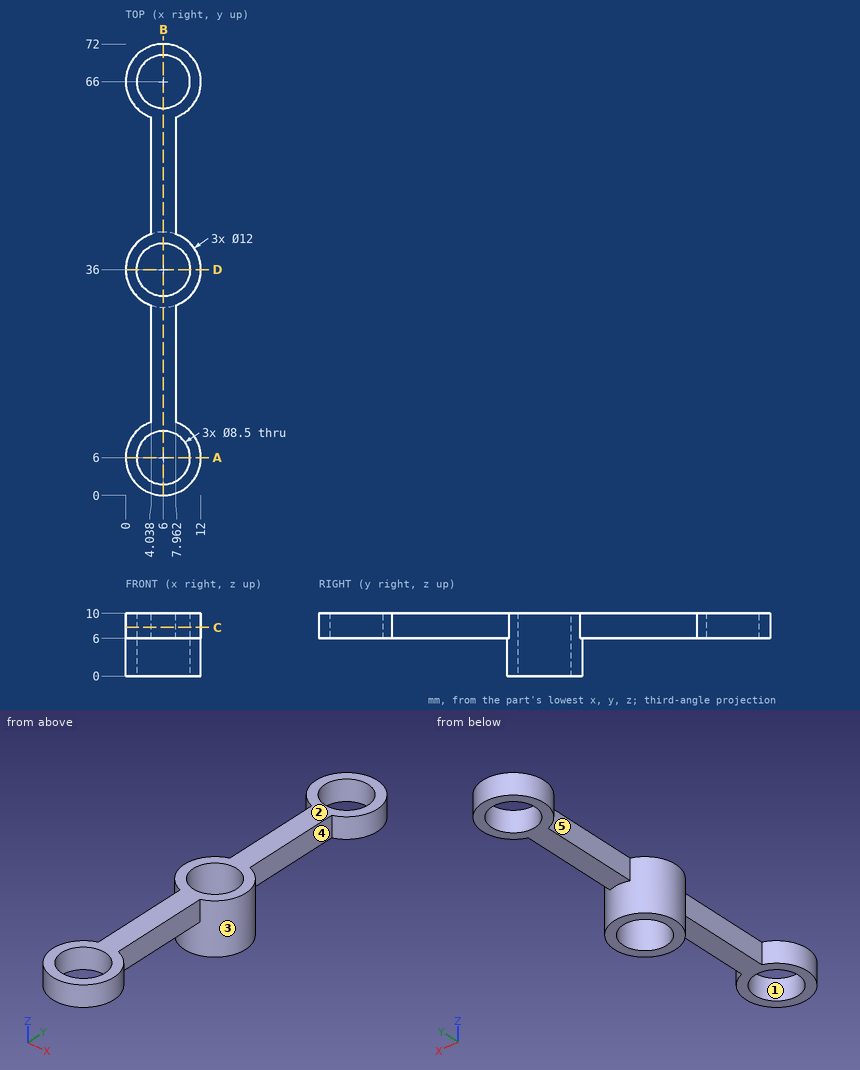
Geometry: see drawing. Coordinates: mm, zero at the bounding-box minimum. A direction names the side the tool comes from. Give positions to 0.01 mm unless a question says otherwise; leave off trailing zeros. Order: outer loops, then holes, each group sorted by start corner. A loop starts at its lowest first (then second) coordinate and runs counter-clockwise, first axis right, second up. Notation, with made-up numbers: M -27,65 L -18,65 A20 cw -18,93 Z; hole C 68.5,47 d4. An arc over 180 degrees is marked long. Answer as a JSON object with one key per item and string values.
1. Cut plane B-B, the plane x = 6. Output: boundary loops of the cut face in (y, z).
Result sheet:
{"outline": "M 0,6 L 1.75,6 L 1.75,10 L 0,10 Z; M 10.25,6 L 30,6 L 30,0 L 31.75,0 L 31.75,10 L 10.25,10 Z; M 40.25,0 L 42,0 L 42,6 L 61.75,6 L 61.75,10 L 40.25,10 Z; M 70.25,6 L 72,6 L 72,10 L 70.25,10 Z"}
2. Cut plane A-A, the plane y = 6. Output: boundary loops of the cut face in (x, z), and give its area (3 significant figures).
Result sheet:
{"outline": "M 0,6 L 1.75,6 L 1.75,10 L 0,10 Z; M 10.25,6 L 12,6 L 12,10 L 10.25,10 Z", "area": "14.0 mm²"}
3. Reachability of the marked faces 3, 4 and 5 from +Z, -Z, +X, -X, +Y, -Y: full face, straight path, thin tool, end or side. Return the list, or none.
Result sheet:
{"face 3": "-Z", "face 4": "+Z, -Z, +X", "face 5": "+Z, -Z, -X"}
4. Ray query, line 1 (X direction, y = 36, z = 4.75); line 2 (Y direction, x = 7.25, z = 7.5); line 3 (Z direction, x = 6.5, y = 59). Return the intervals inside material, ascending. Write a range as [from, to].
Result sheet:
{"line 1": "[0, 1.75], [10.25, 12]", "line 2": "[0.13, 1.94], [10.06, 31.94], [40.06, 61.94], [70.06, 71.87]", "line 3": "[6, 10]"}
5. Cut plane D-D, the plane y = 36. Output: boundary loops of the cut face in (x, z), and give its area (3 significant figures).
Result sheet:
{"outline": "M 0,0 L 1.75,0 L 1.75,10 L 0,10 Z; M 10.25,0 L 12,0 L 12,10 L 10.25,10 Z", "area": "35.0 mm²"}
6. First-contact query: P1, Ø2, axis at y = 25, z = 8.5, coming from the +X side; P2, Ø6, axis at x = 8.5, y = 19.5, coming from the -Z side; P3, Ø6, axis at x = 3, z = 4, coming from the -Y side. Flat tips, straight axial feed; report the tip coordinate or a pass-through.
Result sheet:
{"P1": "x = 7.96", "P2": "z = 6", "P3": "y = 0.05"}
7. Pull-direction query (Y, two-part tool) for the marked faces 1 and 2; classes: +Y half, -Y half, draft (parallel to the pull), parting line (faces both ways), or undercut.
Result sheet:
{"face 1": "undercut", "face 2": "draft"}
8. Cut plane C-C, the plane z = 7.75. Output: boundary loops of the cut face in (x, y).
Result sheet:
{"outline": "M 4.04,11.67 A6 ccw long 7.96,11.67 L 7.96,30.33 A6 ccw 7.96,41.67 L 7.96,60.33 A6 ccw long 4.04,60.33 L 4.04,41.67 A6 ccw 4.04,30.33 Z; hole C 6,6 d8.5; hole C 6,36 d8.5; hole C 6,66 d8.5"}
